Autodesk Inventor part; units mm, degrees
ref_plane "YZ Plane" through (0, 0, 0) normal (1, 0, 0) x (0, 1, 0)
ref_plane "XZ Plane" through (0, 0, 0) normal (0, 1, 0) x (-1, 0, 0)
ref_plane "XY Plane" through (0, 0, 0) normal (0, 0, 1) x (1, 0, 0)
sketch "Inner Rib Profile" plane through (0, 0, 0) normal (1, 0, 0) x (0, 1, 0)
  line L0 (-10, 10) -> (10, 10) construction
  line L1 (10, 10) -> (10, -10) construction
  line L2 (10, -10) -> (-10, -10) construction
  line L3 (-10, -10) -> (-10, 10) construction
  line L4 (-10, 10) -> (10, -10) construction
  line L5 (10, 10) -> (-10, -10) construction
  line L6 (-10, -10) -> (-10, -19)
  line L7 (-10, -19) -> (10, -19)
  line L8 (10, -19) -> (10, -10)
  line L9 (0, 0) -> (-10, 0) construction
  line L10 (-10, 10) -> (-10, 19)
  line L11 (-10, 19) -> (10, 19)
  line L12 (10, 19) -> (10, 10)
  line L13 (-10, 10) -> (-19, 10)
  line L14 (-19, 10) -> (-19, -10)
  line L15 (-19, -10) -> (-10, -10)
  line L16 (0, 0) -> (0, 10) construction
  line L17 (10, 10) -> (19, 10)
  line L18 (19, 10) -> (19, -10)
  line L19 (19, -10) -> (10, -10)
  dimension "d0" = 20
  dimension "d1" = 20
  dimension "d2" = 9
  dimension "d3" = 9
extrude "Make Inner Rib by Extrusion of Its Profile" add sketch "Inner Rib Profile" along normal mid plane 9
sketch "Laser Cutter Sketch" plane through (4.5, 0, 0) normal (1, 0, 0) x (0, 0, -1)
  line L0 (-19, 10) -> (-19, -10) construction
  line L1 (-19, -10) -> (-10, -10) construction
  line L2 (-10, -10) -> (-10, -19)
  line L3 (-10, -19) -> (10, -19)
  line L4 (10, -19) -> (10, -10)
  line L5 (10, -10) -> (19, -10) construction
  line L6 (19, -10) -> (19, 10) construction
  line L7 (19, 10) -> (10, 10) construction
  line L8 (10, 10) -> (10, 19)
  line L9 (10, 19) -> (-10, 19)
  line L10 (-10, 19) -> (-10, 10)
  line L11 (-10, 10) -> (-19, 10) construction
  line L12 (0, 0) -> (0, 19) construction
  line L13 (-5, 0) -> (5, 0) construction
  line L14 (-5, -2.5) -> (5, -2.5)
  line L15 (5, 2.5) -> (-5, 2.5)
  arc A0 (-5, 2.5) -> (-5, -2.5) centre (-5, 0) ccw
  arc A1 (5, -2.5) -> (5, 2.5) centre (5, 0) ccw
  line L16 (10, -10.25) -> (19.25, -10.25)
  line L17 (19.25, -10.25) -> (19.25, 10.25)
  line L18 (19.25, 10.25) -> (10, 10.25)
  line L19 (-10, -10.25) -> (-19.25, -10.25)
  line L20 (-19.25, -10.25) -> (-19.25, 10.25)
  line L21 (-19.25, 10.25) -> (-10, 10.25)
  line L22 (-10, -19) -> (-10, -10.25)
  line L23 (-10, 19) -> (-10, 10.25)
  line L24 (10, -10.25) -> (10, -19)
  line L25 (10, 10.25) -> (10, 19)
  dimension "d7" = 10
  dimension "d8" = 5
  dimension "d13" = 0.25
equation "\"d0\" = InnerRibHeight"
equation "\"d1\" = RibSlotLength"
equation "\"d2\" = PrototypePlateMaterialThickness"
equation "\"d4\" = PrototypePlateRibMaterialThickness"
properties part number "Inner Rib"
Geometry check sheet. Reference: the model listing, model coordinates, mm. A direction names the side the tool comes from. Give positions to 0.01 mm unless a question says otherwise; leave off trailing zeros. Loops run counter-clockwise (first coordinate to the right, second up) from the corner with the lowest first, then second, coordinate; pieces in that order, holes last. Notation, with made-up numbers: M 64,75 L 106,75 A30 cw 106,114 Z; hole C 62,-28 d2. An arc over 180 degrees is marked long. Write each question's results on one line, items separated by ' | '.
1) Section check A-A, the plane x = 1.75. Record the boundary of the cut face in (y, z), plus the area to 3 significant figures.
Answers follow:
outline: M -19,-10 L -10,-10 L -10,-19 L 10,-19 L 10,-10 L 19,-10 L 19,10 L 10,10 L 10,19 L -10,19 L -10,10 L -19,10 Z | area: 1,120 mm2
2) Section check B-B, the plane y = -11.5. Record the boundary of the cut face in (x, z).
Answers follow:
outline: M -4.5,-10 L 4.5,-10 L 4.5,10 L -4.5,10 Z
3) Thickness scan on line 1 (Y direction, x = 2.5, z = 12). Record the ranges inside material, lowest first.
Answers follow:
line 1: -10 to 10
4) Gauge pin test, flat end, axial feed: pin 1 (2.5 mm diameter, centred on x = 0.5, y = 15, fed in from +Z). Record the tip position at first contact, or that the pin passes through.
Answers follow:
pin 1: z = 10
5) Tool access check on faces 1 (the face through (0, 14, 10)), 2 (the face through (0, -15, -10)), 3 (the face through (0, 15, -10)), 4 (the face through (0, -14, 10)), 5 (the face through (0, -19, 0)). Record the directions out of +Z, -Z, +X, -X, +Y, -Y that give a thin tool (end or side, any length) a straight path to the whole face; none if there is none.
Answers follow:
face 1: +Z, +X, -X, +Y | face 2: -Z, +X, -X, -Y | face 3: -Z, +X, -X, +Y | face 4: +Z, +X, -X, -Y | face 5: +Z, -Z, +X, -X, -Y
